Geometry check sheet. Reference: the model listing, model coordinates, mm. Face numbers are marked on the shaded views. Round coordinates to 2 decimals unless told otherwise and drop trailing zeros. Order: outer loops, then holes, each group sorted by start corner. A loop starts at its lowest first (then second) coordinate and runs counter-clockwise, first axis right, second up. Notation, with made-up numbers: (32, -1) - (70, -1) arc R17 cw to (70, 29) - close; hole circle Ø6 at (-6, 22.25). An arc over 180 degrees is marked (long way). Return JSON: item names as keys, results as strings. Group by question number.
Q1. Sectioned sample at A-A, the plane x = 65.5. Record the cut outline in (y, z).
Q2. Sectioned sample at B-B, the plane z = 67.5. Record the cut outline in (x, y), then the cut area to 3 significant figures.
Q3. Sectioned sample at D-D, the plane z = 16. Record the cut outline in (x, y), then the cut area to 3 significant figures.
Q4. Sectioned sample at C-C, the plane y = 7.75. Record the cut outline in (x, z).
Q5. Material ranges on line 1 along Z through (x, y) = (337.5, 14.75); line 2 along Z through (x, y) = (326, 1.5); line 3 along X through (y, z) = (1.3, 80), recorded low to high.
Q6. Draft check along Z on the marked faces 1 and 2. Enter one of: pulls with the +Z half, pulls with the -Z half, needs draft (parallel to the pull), parting line crosses it, or undercut.
Q7. Gauge pin test, flat ends, axial feed: pin 1 Ø20 at (x, z) = (114, 88) entering from +Y; pin 2 Ø12 at (y, z) = (14.5, -76.5) entering from -X; pin 3 Ø10 at (x, y) = (176, 9) entering from +Z; pin 4 Ø3 at (x, z) = (90.5, -46) entering from +Y. Record the tip position at first contact, or that the pin passes through.
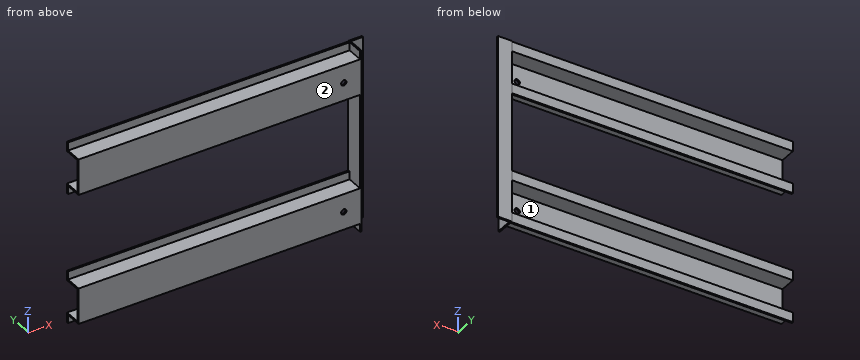
```python
from build123d import *

# Parameters (mm, degrees)
EXTRUDE_THIN1_DEPTH     = 346
SKETCH5_R               = 3.3
CUT_EXTRUDE1_DEPTH      = 365.225205059
CUT_EXTRUDE1_DEPTH_BACK = 365.225205059
SKETCH6_W               = 23
SKETCH6_H               = 224
BOSS_EXTRUDE2_DEPTH     = 2
SKETCH8_W               = 2
SKETCH8_H               = 224
EXTRUDE_THIN2_DEPTH     = 15


with BuildPart() as part:
    # Sketch2 → Extrude-Thin1 (new body)
    with BuildSketch(Plane.YZ):
        Polygon((20, 112), (20, 102), (0, 102), (0, 58), (20, 58), (20, 48), (22, 48), (22, 60), (2, 60), (2, 100), (22, 100), (22, 112), align=None)
    extrude(amount=-EXTRUDE_THIN1_DEPTH)

    # Sketch5 → Cut-Extrude1 (cut, two sides)
    with BuildSketch(Plane(origin=(0, 2, 0), x_dir=(-1, 0, 0), z_dir=(0, 1, 0))) as cut_extrude1_sk:
        with Locations(Location((326, 80, 0), (0, 0, 90))):
            Circle(SKETCH5_R)
    extrude(amount=CUT_EXTRUDE1_DEPTH, mode=Mode.SUBTRACT)
    extrude(cut_extrude1_sk.sketch, amount=-CUT_EXTRUDE1_DEPTH_BACK, mode=Mode.SUBTRACT)


with BuildPart() as body_2:
    # Mirror1: mirrored copy
    add(part.part.mirror(Plane.XY))


with BuildPart() as part_1:
    add(part.part)

    add(body_2.part)  # Boss-Extrude2 merges body 2
    # Sketch6 → Boss-Extrude2 (add)
    with BuildSketch(Plane(origin=(-346, 0, 0), x_dir=(0, 1, 0), z_dir=(-1, 0, 0))):
        with Locations((11.5, 0)):
            Rectangle(SKETCH6_W, SKETCH6_H)
    extrude(amount=BOSS_EXTRUDE2_DEPTH)

    # Sketch8 → Extrude-Thin2 (add)
    with BuildSketch(Plane(origin=(-348, 0, 0), x_dir=(0, -1, 0), z_dir=(-1, 0, 0))):
        with Locations((-22, 0)):
            Rectangle(SKETCH8_W, SKETCH8_H)
    extrude(amount=EXTRUDE_THIN2_DEPTH)

    # Mirror2: part across plane


with BuildPart() as part_2:
    add(part_1.part)
    add(part_1.part.mirror(Plane(origin=(0, 0, 0), x_dir=(0, 0, 1), z_dir=(1, 0, 0))))

    # SurfaceCut1
    split(bisect_by=Plane.YZ, keep=Keep.TOP)


solid = part_2.part
```
Reply:
{
 "1": {"outline": "(0, -102) - (20, -102) - (20, -112) - (22, -112) - (22, -100) - (2, -100) - (2, -60) - (22, -60) - (22, -48) - (20, -48) - (20, -58) - (0, -58) - close; (0, 58) - (20, 58) - (20, 48) - (22, 48) - (22, 60) - (2, 60) - (2, 100) - (22, 100) - (22, 112) - (20, 112) - (20, 102) - (0, 102) - close"},
 "2": {"outline": "(0, 0) - (348, 0) - (348, 21) - (363, 21) - (363, 23) - (346, 23) - (346, 2) - (0, 2) - close", "area": "768 mm^2"},
 "3": {"outline": "(346, 0) - (348, 0) - (348, 21) - (363, 21) - (363, 23) - (346, 23) - close", "area": "76.0 mm^2"},
 "4": {"outline": "(0, -102) - (346, -102) - (346, -112) - (348, -112) - (348, 112) - (346, 112) - (346, 102) - (0, 102) - (0, 100) - (346, 100) - (346, 60) - (0, 60) - (0, 58) - (346, 58) - (346, -58) - (0, -58) - (0, -60) - (346, -60) - (346, -100) - (0, -100) - close"},
 "5": {"line 1": "-102 to -100, -60 to -58, 58 to 60, 100 to 102", "line 2": "-102 to -83.3, -76.7 to -58, 58 to 76.7, 83.3 to 102", "line 3": "0 to 322.7, 329.3 to 348"},
 "6": {"face 1": "undercut", "face 2": "needs draft"},
 "7": {"pin 1": "y = 2", "pin 2": "x = 346", "pin 3": "z = 102", "pin 4": "through"}
}
